Print and shaded views of the part. All mm, measured from the part's lowest x, y and z. Coordinates: 2 decimals unless noted, no trailing zeros. Loops run counter-clockwise (first coordinate to the right, second up) from the corner with the lowest first, then second, coordinate; pieces in that order, holes last. Notation, with made-up numbers: M -32,79 L -12,79 A36 cw -12,116 Z; hole C 66.5,-18 d1. An arc over 180 degrees is marked long. Answer as a JSON object with one key per item and string values. Group by question number.
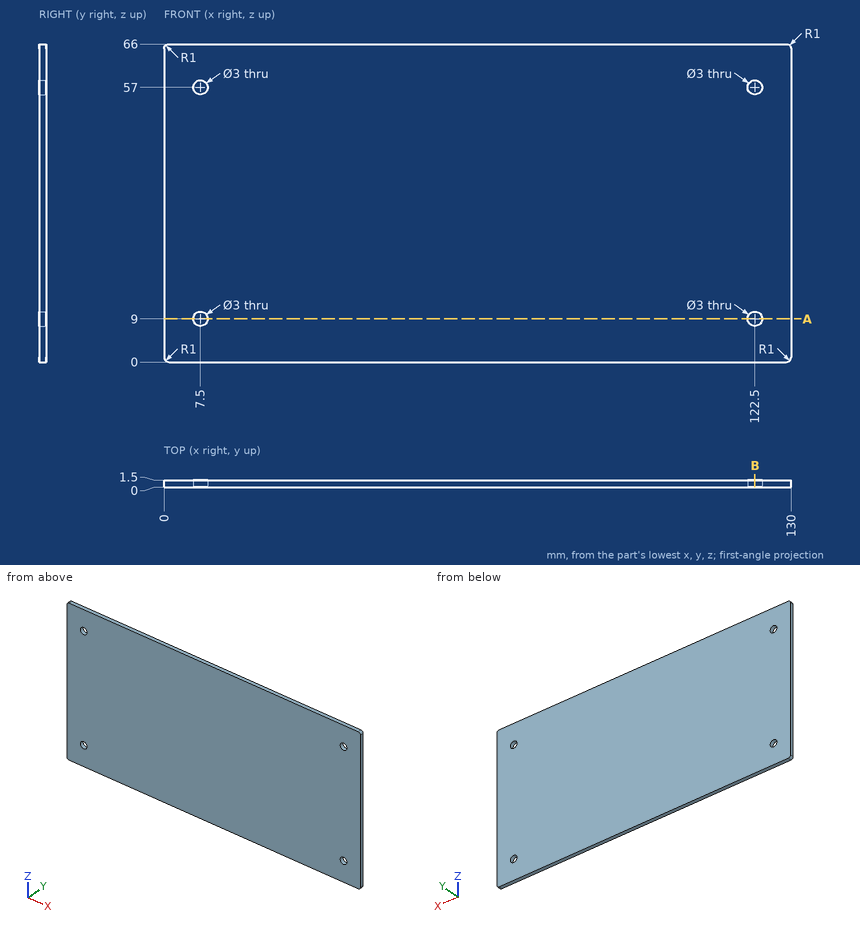
Item 1: Slice it at B-B, the plane x = 122.5. Write the cut outline in (y, z).
Item 2: Slice it at A-A, the plane z = 9. Write the cut outline in (x, y), then the cut area to 3 significant figures.
Item 3: Drill centre lines: L1, parallel to X at y = 0.9, z = 9; L2, parallel to X at y = 0.1, z = 58; L3, parallel to Z at x = 123, y = 0.3. Where is each one in solid material? Low to high. Write a range as from..to.
Computed:
{
 "1": {"outline": "M 0,0 L 1.5,0 L 1.5,7.5 L 0,7.5 Z; M 0,10.5 L 1.5,10.5 L 1.5,55.5 L 0,55.5 Z; M 0,58.5 L 1.5,58.5 L 1.5,66 L 0,66 Z"},
 "2": {"outline": "M 0,0 L 6,0 L 6,1.5 L 0,1.5 Z; M 9,0 L 121,0 L 121,1.5 L 9,1.5 Z; M 124,0 L 130,0 L 130,1.5 L 124,1.5 Z", "area": "186 mm2"},
 "3": {"L1": "0..6, 9..121, 124..130", "L2": "0..6.38, 8.62..121.38, 123.62..130", "L3": "0..7.59, 10.41..55.59, 58.41..66"}
}
